For this review, take the finished solid that the model builds, in its own axes (mm). A direction names the side the tool comes from. Coordinates: 2 decimals unless noted, no trailing zeros. Write each loop counter-clockwise with the first axis right and the second up, starting at its lowest first coordinate (ties: lowest second). Pieces come first, ordered by that corner, then holes. Notation, with made-up numbers: (47, 36) -> (61, 36) arc R37 cw to (61, 74) -> close; hole circle Ø8 at (32, -39). An arc over 180 degrees is marked (long way). One line per item, written item: value. Start each with the question number.
1) Machinability: for faces 1 (the conical face through (-13.096, -25.178, -23.9)), 2 (the conical face through (-2.01, 9.05, -43.51)), 3 (the cylindrical face through (-31, 9.76, -10.09)), which of the approach directions +Z, -Z, +X, -X, +Y, -Y give a long, thin tool a straight path to every point of the face, cutting with its end or side? Answer none if there is none.
2) Add section A-A (x = 0). State the section outline as (y, z) points.
3) For pin 1 Ø10 at (x, z) = (-15, -24.5) entering from +Y; pin 2 Ø4 at (x, y) = (32.5, -43.5) entering from -Z; pin 3 Ø5 at (y, z) = (-34, -55.5) entering from -X; pin 4 Ø1 at (x, y) = (30.5, 10) entering from +Z, all flat-tipped, find the tip position at first contact; note any pin that passes through.
4) For probe 1 along Y at (x, z) = (0, -11); probe 2 along Y at (x, z) = (0, -29.5); probe 3 along X at (y, z) = (1.5, -2.5), list the stretches that pass through material, from the lowest coordinate up. Write a range as from..to.
5) Mouldability with a two-part tool opening along X and no side actions: class faces 4 (the flat face through (-5, -5, 0.735)), 5 (the conical face through (5.521, -24.864, 0.465)), 6 (the cylindrical face through (5.96, 1.88, -20.4)) as released by +X, released by -X, zero draft, split by the parting line, or undercut.
6) Add section D-D (z = -15). State the section outline as (x, y) points.
7) Add section C-C (z = -33.5). State the section outline as (x, y) points, and give its area (3 significant figures).
from build123d import *

# Parameters (mm, degrees)
SKETCH56_R           = 6.5
BOSS_EXTRUDE10_DEPTH = 5
CHAMFER1_SIZE        = 1.5
CHAMFER1_SIZE2       = 0.866025404
CHAMFER2_SIZE        = 1.5
CHAMFER2_SIZE2       = 0.866025404
SKETCH59_R           = 5.633974596
BOSS_EXTRUDE12_DEPTH = 3
SKETCH60_R           = 5.5
BOSS_EXTRUDE13_DEPTH = 5
BOSS_EXTRUDE13_DRAFT = -50
SKETCH64_R           = 1.25
CUT_EXTRUDE3_DEPTH   = 53
FILLET3_R            = 0.5
SCALE1_SCALE         = 5


with BuildPart() as part:
    # Sketch56 → Boss-Extrude10 (new body)
    with BuildSketch(Plane(origin=(0, 0, -24.5), x_dir=(-1, 0, 0), z_dir=(0, 0, -1))):
        Circle(SKETCH56_R)
    extrude(amount=BOSS_EXTRUDE10_DEPTH)

    # Chamfer1
    chamfer1_edges = [part.edges().sort_by_distance(p)[0] for p in [
        (6.5, 0, -24.5),
    ]]
    chamfer1_side = [part.faces().sort_by_distance(p)[0] for p in [
        (0, 0, -24.5),
    ]]
    chamfer(chamfer1_edges, length=CHAMFER1_SIZE, length2=CHAMFER1_SIZE2, reference=chamfer1_side[0])

    # Chamfer2
    chamfer2_edges = [part.edges().sort_by_distance(p)[0] for p in [
        (6.5, 0, -29.5),
    ]]
    chamfer2_side = [part.faces().sort_by_distance(p)[0] for p in [
        (6.5, 0, -27.433012702),
    ]]
    chamfer(chamfer2_edges, length=CHAMFER2_SIZE, length2=CHAMFER2_SIZE2, reference=chamfer2_side[0])

    # Sketch59 → Boss-Extrude12 (add)
    with BuildSketch(Plane(origin=(0, 0, -29.5), x_dir=(-1, 0, 0), z_dir=(0, 0, -1))):
        with Locations(Location((0, 0, 0), (0, 0, 180))):
            Circle(SKETCH59_R)
    extrude(amount=BOSS_EXTRUDE12_DEPTH)


with BuildPart() as boss_extrude13_tool:
    # Sketch60 → Boss-Extrude13 (with draft: the straight prism first)
    with BuildSketch(Plane(origin=(0, 0, -32.5), x_dir=(-1, 0, 0), z_dir=(0, 0, -1))):
        Circle(SKETCH60_R)
    extrude(amount=BOSS_EXTRUDE13_DEPTH)
    # Boss-Extrude13: the draft: its side faces are tilted about the plane it starts from
    boss_extrude13_sides = [boss_extrude13_tool.faces().sort_by_distance(p)[0] for p in [
        (5.5, 0, -35),
    ]]
    draft(boss_extrude13_sides, Plane(origin=(0, 0, -32.5), x_dir=(-1, 0, 0), z_dir=(0, 0, -1)), BOSS_EXTRUDE13_DRAFT)


with BuildPart() as part_1:
    add(part.part)

    # Boss-Extrude13: add boss_extrude13_tool
    add(boss_extrude13_tool.part)

    # Sketch62 → Cut-Revolve2 (revolve, cut)
    with BuildSketch(Plane(origin=(0, 0, 0), x_dir=(0, 0, -1), z_dir=(1, 0, 0)), mode=Mode.PRIVATE) as cut_revolve2_sk:
        Polygon((32.5, 0), (37.5, 10.922090923), (37.5, 0), align=None)
    revolve(cut_revolve2_sk.sketch.rotate(Axis((0, 0, -32.5), (0, 0, -1)), 90), axis=Axis((0, 0, -32.5), (0, 0, -1)), mode=Mode.SUBTRACT)

    # Sketch64 → Cut-Extrude3 (cut)
    with BuildSketch(Plane.XY.offset(-24.5)):
        Circle(SKETCH64_R)
    extrude(amount=-CUT_EXTRUDE3_DEPTH, mode=Mode.SUBTRACT)

    # Fillet3
    # the kernel refuses this fillet: 0.5 mm, written as the material it takes off along each edge
    with BuildSketch(Plane(origin=(0, 0, -32.5), x_dir=(1, 0, 0), z_dir=(0, 1, 0))) as fillet3_piece_1:
        with BuildLine():
            CenterArc((5.133974596, -0.340625019), FILLET3_R, 0, 42.941402865)
            Line((5.5, 0), (5.633974596, 0))
            Line((5.633974596, 0), (5.633974596, -0.340625019))
        make_face()
    revolve(axis=Axis((0, 0, -32.5), (0, 0, -1)), mode=Mode.SUBTRACT)


with BuildPart() as part_2:
    # Scale1: scaled about (0, 0, -30.8088706)
    add(part_1.part.scale(SCALE1_SCALE).moved(Location((0, 0, 123.2354824))))


solid = part_2.part
Numbers:
1. face 1: none
1. face 2: -Z
1. face 3: +Z
2. outline: (-57.29, -64.26) -> (-54.61, -64.26) -> (-6.25, -42.13) -> (-6.25, 0.74) -> (-25, 0.74) -> (-32.5, -3.59) -> (-32.5, -16.76) -> (-28.17, -24.26) -> (-28.17, -37.56) arc R2.5 ccw to (-27.5, -39.26) -> close; (6.25, -42.13) -> (54.61, -64.26) -> (57.29, -64.26) -> (27.5, -39.26) arc R2.5 ccw to (28.17, -37.56) -> (28.17, -24.26) -> (32.5, -16.76) -> (32.5, -3.59) -> (25, 0.74) -> (6.25, 0.74) -> close
3. pin 1: y = 27.87
3. pin 2: z = -64.26
3. pin 3: x = -37.02
3. pin 4: z = -3.07
4. probe 1: -32.5..-6.25, 6.25..32.5
4. probe 2: -28.17..-6.25, 6.25..28.17
4. probe 3: -30.57..-6.07, 6.07..30.57
5. face 4: zero draft
5. face 5: split by the parting line
5. face 6: undercut
6. outline: circle Ø65 at (0, 0); hole circle Ø12.5 at (0, 0)
7. outline: circle Ø56.34 at (0, 0); hole circle Ø12.5 at (0, 0)
7. area: 2,370 mm²
